Source: CAD feature listing. Evaluate the final solid. Frame: model axes, mm. Face numbers are marked on the shaded views. A direction names the side the tool comes from. Coordinates: 2 decimals unless noted, no trailing zeros. Loops run counter-clockwise (first coordinate to the right, second up) from the corner with the lowest first, then second, coordinate; pieces in that order, holes last. Notation, with made-up numbers: (21.5, 68) - (63.5, 68) arc R23 ccw to (63.5, 89) - close; hole circle Ø8 at (50.25, -9.75). An arc over 180 degrees is marked (long way). Use one line per item in the form item = value. Start each with the question number.
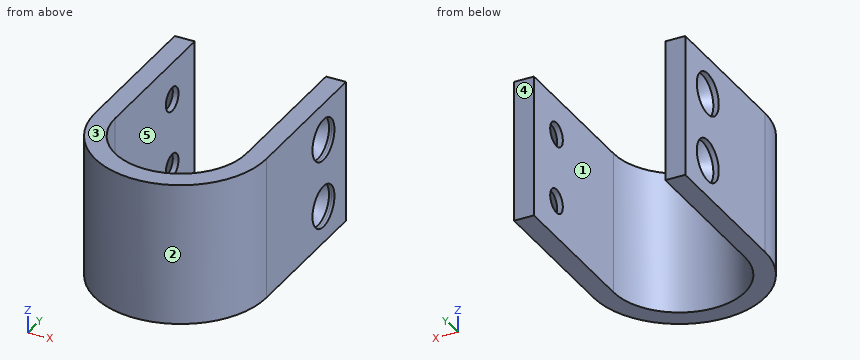
from build123d import *

# Parameters (mm, degrees)
EXTRUDE_1391_DEPTH               = 25
CUT_EXTRUDE_1919_REACH           = 49.194
SKETCH_1505_R                    = 2.1
SKETCH_2_3_R                     = 3.65
SKETCH_2_3_R_2                   = 2.1
CUT_EXTRUDE_1959_DEPTH           = 0.5
CHAMFER_2009_SIZE                = 2
CHAMFER_2009_OF_MIRROR_2081_SIZE = 2


with BuildPart() as part:
    # Sketch 313 → Extrude 1391 (new body)
    with BuildSketch(Plane.XY):
        with BuildLine():
            Line((-11.5, 0), (-11.5, 26.5))
            Line((-11.5, 26.5), (-15, 26.5))
            Line((-15, 26.5), (-15, 0))
            ThreePointArc((-15, 0), (0, -15), (15, 0))
            Line((15, 0), (15, 26.5))
            Line((15, 26.5), (11.5, 26.5))
            Line((11.5, 26.5), (11.5, 0))
            ThreePointArc((11.5, 0), (0, -11.5), (-11.5, 0))
        make_face()
    extrude(amount=EXTRUDE_1391_DEPTH)

    # Sketch 1505 → Cut-Extrude 1919 (cut, up to next)
    with BuildSketch(Plane.ZY.offset(15), mode=Mode.PRIVATE) as cut_extrude_1919_sk1:
        with Locations((6.5, 19)):
            Circle(SKETCH_1505_R)
    cut_extrude_1919_tool1 = extrude(cut_extrude_1919_sk1.sketch, amount=-CUT_EXTRUDE_1919_REACH, mode=Mode.PRIVATE) & part.part
    # Sketch 1505 → Cut-Extrude 1919 (cut, up to next)
    with BuildSketch(Plane.ZY.offset(15), mode=Mode.PRIVATE) as cut_extrude_1919_sk2:
        with Locations((18.5, 19)):
            Circle(SKETCH_1505_R)
    cut_extrude_1919_tool2 = extrude(cut_extrude_1919_sk2.sketch, amount=-CUT_EXTRUDE_1919_REACH, mode=Mode.PRIVATE) & part.part
    cut_extrude_1919_1 = cut_extrude_1919_tool1.solids().sort_by_distance((-15, 19, 6.5))[0]
    add(cut_extrude_1919_1, mode=Mode.SUBTRACT)
    cut_extrude_1919_2 = cut_extrude_1919_tool2.solids().sort_by_distance((-15, 19, 18.5))[0]
    add(cut_extrude_1919_2, mode=Mode.SUBTRACT)
    cut_extrude_1919 = cut_extrude_1919_1 + cut_extrude_1919_2  # Cut-Extrude 1919 as one shape, for the pattern or mirror that repeats it

    # Эскиз2<3> → Cut-Extrude 1959 (cut)
    # profile 1 of 2: a face of its own
    with BuildSketch(Plane.ZY.offset(15)):
        with Locations((6.5, 19)):
            Circle(SKETCH_2_3_R)
        with Locations((6.5, 19)):
            Circle(SKETCH_2_3_R_2, mode=Mode.SUBTRACT)
    # profile 2 of 2: a face of its own
    with BuildSketch(Plane.ZY.offset(15)):
        with Locations(Location((18.5, 19, 0), (0, 0, 180))):
            Circle(SKETCH_2_3_R)
        with Locations((18.5, 19)):
            Circle(SKETCH_2_3_R_2, mode=Mode.SUBTRACT)
    cut_extrude_1959 = extrude(amount=-CUT_EXTRUDE_1959_DEPTH, mode=Mode.SUBTRACT)

    # Chamfer 2009
    # the kernel refuses this chamfer: 2 mm, written as the material it takes off along each edge
    with BuildSketch(Plane(origin=(-14.5, 19, 18.5), x_dir=(0, 0, 1), z_dir=(0, -1, 0))) as chamfer_2009_piece_1_section:
        Polygon((2.1, -CHAMFER_2009_SIZE), (2.1 + CHAMFER_2009_SIZE, 0), (2.1, 0), align=None)
    chamfer_2009_piece_1 = revolve(axis=Axis((-14.5, 19, 18.5), (-1, 0, 0)), mode=Mode.PRIVATE)
    chamfer_2009_piece_1 = chamfer_2009_piece_1 & Plane(origin=(-13.269804267, 19, 18.5), x_dir=(0, 0, -1), z_dir=(-1, 0, 0)) * Cylinder(3.65, 17, mode=Mode.PRIVATE)
    add(chamfer_2009_piece_1, mode=Mode.SUBTRACT)
    with BuildSketch(Plane(origin=(-14.5, 19, 6.5), x_dir=(0, 0, 1), z_dir=(0, -1, 0))) as chamfer_2009_piece_2_section:
        Polygon((2.1, -CHAMFER_2009_SIZE), (2.1 + CHAMFER_2009_SIZE, 0), (2.1, 0), align=None)
    chamfer_2009_piece_2 = revolve(axis=Axis((-14.5, 19, 6.5), (-1, 0, 0)), mode=Mode.PRIVATE)
    chamfer_2009_piece_2 = chamfer_2009_piece_2 & Plane(origin=(-13.269804267, 19, 6.5), x_dir=(0, 0, 1), z_dir=(-1, 0, 0)) * Cylinder(3.65, 17, mode=Mode.PRIVATE)
    add(chamfer_2009_piece_2, mode=Mode.SUBTRACT)

    # Mirror 2081: Cut-Extrude 1919, Cut-Extrude 1959 across plane
    add(cut_extrude_1919.mirror(Plane(origin=(0, 0, 0), x_dir=(0, 0, 1), z_dir=(1, 0, 0))), mode=Mode.SUBTRACT)
    add(cut_extrude_1959.mirror(Plane(origin=(0, 0, 0), x_dir=(0, 0, 1), z_dir=(1, 0, 0))), mode=Mode.SUBTRACT)

    # Chamfer 2009 of Mirror 2081
    # the kernel refuses this chamfer: 2 mm, written as the material it takes off along each edge
    with BuildSketch(Plane(origin=(14.5, 19, 18.5), x_dir=(0, 0, 1), z_dir=(0, -1, 0))) as chamfer_2009_of_mirror_2081_piece_1_section:
        Polygon((2.1, CHAMFER_2009_OF_MIRROR_2081_SIZE), (2.1 + CHAMFER_2009_OF_MIRROR_2081_SIZE, 0), (2.1, 0), align=None)
    chamfer_2009_of_mirror_2081_piece_1 = revolve(axis=Axis((14.5, 19, 18.5), (-1, 0, 0)), mode=Mode.PRIVATE)
    chamfer_2009_of_mirror_2081_piece_1 = chamfer_2009_of_mirror_2081_piece_1 & Plane(origin=(13.269804267, 19, 18.5), x_dir=(0, 0, -1), z_dir=(1, 0, 0)) * Cylinder(3.65, 17, mode=Mode.PRIVATE)
    add(chamfer_2009_of_mirror_2081_piece_1, mode=Mode.SUBTRACT)
    with BuildSketch(Plane(origin=(14.5, 19, 6.5), x_dir=(0, 0, 1), z_dir=(0, -1, 0))) as chamfer_2009_of_mirror_2081_piece_2_section:
        Polygon((2.1, CHAMFER_2009_OF_MIRROR_2081_SIZE), (2.1 + CHAMFER_2009_OF_MIRROR_2081_SIZE, 0), (2.1, 0), align=None)
    chamfer_2009_of_mirror_2081_piece_2 = revolve(axis=Axis((14.5, 19, 6.5), (-1, 0, 0)), mode=Mode.PRIVATE)
    chamfer_2009_of_mirror_2081_piece_2 = chamfer_2009_of_mirror_2081_piece_2 & Plane(origin=(13.269804267, 19, 6.5), x_dir=(0, 0, 1), z_dir=(1, 0, 0)) * Cylinder(3.65, 17, mode=Mode.PRIVATE)
    add(chamfer_2009_of_mirror_2081_piece_2, mode=Mode.SUBTRACT)


solid = part.part
(1) Material intervals for line 1 (Z direction, x = 14.35, y = 19); line 2 (X direction, y = 9, z = 7.5); line 3 (X direction, y = -9.5, z = 16), sorted ascending.
(2) Cut plane A-A, the plane z = 6.5. Output: boundary loops of the cut face in (x, y).
(3) Contact query for flat-ended pins moving along their axis: pin 1 (4.5 mm diameter, centred on y = 19, z = 18.5, fed in from -X); pin 2 (6 mm diameter, centred on y = 19, z = 6.5, fed in from -X); pin 3 (3 mm diameter, centred on x = 9.5, z = 3.5, fed in from -Y). Output: stop coordinate, or through.
(4) Cut plane D-D, the plane x = 13. Output: boundary loops of the cut face in (y, z).
(5) Mould query, pull axis X, two halves, no side actions, for the marked faces 1, 2 and 3. Classes: +X half, -X half, draft (parallel to the pull), parting line (faces both ways), or undercut.
(6) Cut plane B-B, the plane y = 24. Output: boundary loops of the cut face in (x, z).
(7) Access query for the marked faces 4 and 5. Directions: +Z, -Z, +X, -X, +Y, -Y. A direction counts if a zero-diameter tool reaches every point of the face in a straight line with its end or side. Return the directions, or none.
(8) Cut plane C-C, the plane z = 12.75. Output: boundary loops of the cut face in (x, y), plus the area to 3 significant figures.
Recorded:
q1.line_1 = 0 to 2.85, 10.15 to 14.85, 22.15 to 25
q1.line_2 = -15 to -11.5, 11.5 to 15
q1.line_3 = -11.61 to -6.48, 6.48 to 11.61
q2.outline = (-15, 0) arc R15 ccw to (15, 0) - (15, 15.35) - (14.05, 15.35) - (12.5, 16.9) - (11.5, 16.9) - (11.5, 0) arc R11.5 cw to (-11.5, 0) - (-11.5, 16.9) - (-12.5, 16.9) - (-14.05, 15.35) - (-15, 15.35) - close; (-15, 22.65) - (-14.05, 22.65) - (-12.5, 21.1) - (-11.5, 21.1) - (-11.5, 26.5) - (-15, 26.5) - close; (11.5, 21.1) - (12.5, 21.1) - (14.05, 22.65) - (15, 22.65) - (15, 26.5) - (11.5, 26.5) - close
q3.pin_1 = -12.65
q3.pin_2 = -13.4
q3.pin_3 = -12.69
q4.outline = (-7.48, 0) - (26.5, 0) - (26.5, 25) - (-7.48, 25) - close; hole circle Ø5.2 at (19, 6.5); hole circle Ø5.2 at (19, 18.5)
q5.face_1 = undercut
q5.face_2 = parting line
q5.face_3 = draft
q6.outline = (-15, 0) - (-11.5, 0) - (-11.5, 25) - (-15, 25) - close; (11.5, 0) - (15, 0) - (15, 25) - (11.5, 25) - close
q7.face_4 = +Z, -Z, +X, -X, +Y
q7.face_5 = +Z, -Z, +Y
q8.outline = (-15, 0) arc R15 ccw to (15, 0) - (15, 26.5) - (11.5, 26.5) - (11.5, 0) arc R11.5 cw to (-11.5, 0) - (-11.5, 26.5) - (-15, 26.5) - close
q8.area = 331 mm²
